Could you check a few things on this model? Use its own coordinates, in mm. Face numbers are marked on the shaded views. A direction names the side the tool comes from. Coordinates: 2 decimals unless noted, no trailing zeros. Write each loop counter-clockwise with the first axis right and the second up, starting at its lowest first coordinate (ties: lowest second). Pieces come first, ordered by that corner, then holes.
```python
from build123d import *

# Parameters (mm, degrees)
SKETCH1_R           = 177.8
BOSS_EXTRUDE2_DEPTH = 1092.2


with BuildPart() as part:
    # Sketch1 → Boss-Extrude2 (new body)
    with BuildSketch(Plane.XY):
        with BuildLine():
            Line((-355.6, 279.4), (-355.6, -177.8))
            Line((-355.6, -177.8), (-177.8, -355.6))
            Line((-177.8, -355.6), (0, -355.6))
            Line((0, -355.6), (535.092306886, -355.6))
            ThreePointArc((535.092306886, -355.6), (618.029295725, -386.420709701), (660.711530918, -463.923529412))
            ThreePointArc((660.711530918, -463.923529412), (720.067018079, -663.338070349), (832.816911878, -838.2))
            Line((832.816911878, -838.2), (965.2, -838.2))
            Line((965.2, -838.2), (1701.8, 0))
            Line((1701.8, 0), (1701.8, 482.6))
            Line((1701.8, 482.6), (1574.8, 609.6))
            Line((1574.8, 609.6), (838.2, 609.6))
            ThreePointArc((838.2, 609.6), (625.746325122, 428.755865672), (348.709613385, 395.713086728))
            Line((348.709613385, 395.713086728), (0, 457.2))
            Line((0, 457.2), (-177.8, 457.2))
            Line((-177.8, 457.2), (-355.6, 279.4))
        make_face()
        Circle(SKETCH1_R, mode=Mode.SUBTRACT)
    extrude(amount=BOSS_EXTRUDE2_DEPTH)


solid = part.part
```
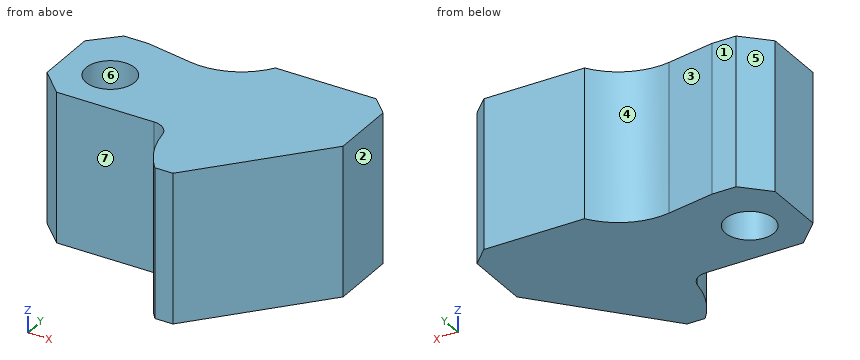
1. I want a section at B-B on x = 87. Please give me the cut outline in (y, z).
Verdict:
outline: (-355.6, 0) - (-155.06, 0) - (-155.06, 1092.2) - (-355.6, 1092.2) - close; (155.06, 0) - (441.86, 0) - (441.86, 1092.2) - (155.06, 1092.2) - close
2. For pin 1 (10 mm diameter, centred on x = 293, z = 581.5, fed in from +Y); pin 2 (3 mm diameter, centred on x = 999.5, z = 922.5, fed in from -Y); pin 3 (8 mm diameter, centred on x = -109, z = 316.5, fed in from +Y); pin 4 (12 mm diameter, centred on x = 1059.5, y = 345, fed in from -Z), each with a flat end and sliding along its axis, tell me the tip position at first contact or that it passes through.
Verdict:
pin 1: stops at y = 406.42
pin 2: stops at y = -800.88
pin 3: stops at y = 457.2
pin 4: stops at z = 0
3. I want a section at C-C on y = 505. Please give me the cut outline in (x, z), plus the area to 3 significant figures.
Verdict:
outline: (747.09, 0) - (1679.4, 0) - (1679.4, 1092.2) - (747.09, 1092.2) - close
area: 1,020,000 mm2
4. If we mould it in two halves opening along X, with no side actions, what happens to the marked faces 4, 5, 6 and 7? For each: pulls with the +X half, pulls with the -X half, needs draft (parallel to the pull), parting line crosses it, or undercut.
Verdict:
face 4: undercut
face 5: pulls with the -X half
face 6: undercut
face 7: needs draft
5. On a 3-axis mill with a long thin cutter (end or side, diameter ignored), from which of +Z, -Z, +X, -X, +Y, -Y can I reach the whole of each face in a straight line? I mean the marked faces 1, 2 and 3. Say none if no direction works.
Verdict:
face 1: +Z, -Z, -X, +Y
face 2: +Z, -Z, +X, +Y, -Y
face 3: +Z, -Z, +Y
6. Please list where these lines run through material, in increasing order: line 1 along Y through (x, z) = (0, 583); line 2 along X through (y, z) = (128.5, 123.5); line 3 along Y through (x, z) = (-62, 809.5).
Verdict:
line 1: y = -355.6 to -177.8, 177.8 to 457.2
line 2: x = -355.6 to -122.88, 122.88 to 1701.8
line 3: y = -355.6 to -166.64, 166.64 to 457.2
7. I want a section at D-D on x = 609. Please give me the cut outline in (y, z).
Verdict:
outline: (-379.32, 0) - (421.81, 0) - (421.81, 1092.2) - (-379.32, 1092.2) - close
8. I want a section at A-A on z = 768.5. Please give me the cut outline in (x, y), plus the area to 3 significant figures.
Verdict:
outline: (-355.6, -177.8) - (-177.8, -355.6) - (535.09, -355.6) arc R127 cw to (660.71, -463.92) arc R736.6 ccw to (832.82, -838.2) - (965.2, -838.2) - (1701.8, 0) - (1701.8, 482.6) - (1574.8, 609.6) - (838.2, 609.6) arc R482.6 cw to (348.71, 395.71) - (0, 457.2) - (-177.8, 457.2) - (-355.6, 279.4) - close; hole circle Ø355.6 at (0, 0)
area: 1,820,000 mm2
